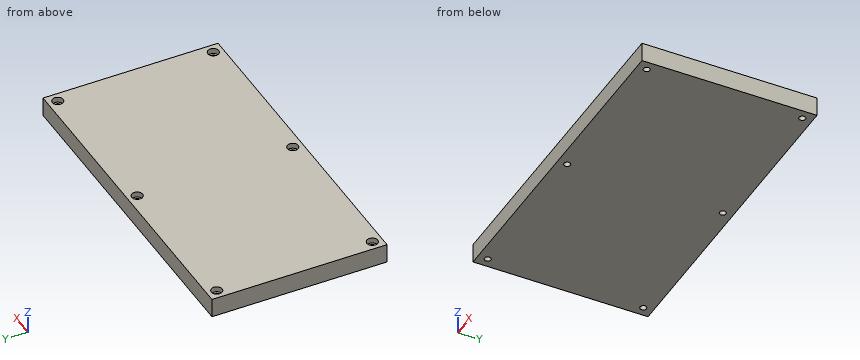
from build123d import *

# Parameters (mm, degrees)
SKETCH1_W                                      = 169.5
SKETCH1_H                                      = 90
BOSS_EXTRUDE1_DEPTH                            = 10
CBORE_FOR_4_SOCKET_HEAD_CAP_SCREW1_D           = 3.2639
CBORE_FOR_4_SOCKET_HEAD_CAP_SCREW1_CBORE_D     = 5.55752
CBORE_FOR_4_SOCKET_HEAD_CAP_SCREW1_CBORE_DEPTH = 2.8448


with BuildPart() as part:
    # Sketch1 → Boss-Extrude1 (new body)
    with BuildSketch(Plane.XY):
        with Locations((84.75, 45)):
            Rectangle(SKETCH1_W, SKETCH1_H)
    extrude(amount=BOSS_EXTRUDE1_DEPTH)

    # CBORE for #4 Socket Head Cap Screw1 (through all)
    with Locations(Plane.XY.offset(10)):
        with Locations((5, 85), (164.5, 85), (164.5, 5), (5, 5), (84.75, 5), (84.75, 85)):
            CounterBoreHole(CBORE_FOR_4_SOCKET_HEAD_CAP_SCREW1_D / 2, CBORE_FOR_4_SOCKET_HEAD_CAP_SCREW1_CBORE_D / 2, CBORE_FOR_4_SOCKET_HEAD_CAP_SCREW1_CBORE_DEPTH)


solid = part.part
Verification items for the finished model (mm, model axes). Coordinates: 2 decimals unless noted, no trailing zeros. Order: outer loops, then holes, each group sorted by start corner. A loop starts at its lowest first (then second) coordinate and runs counter-clockwise, first axis right, second up. Notation, with made-up numbers: M -9.5,10.25 L 25.5,10.25 A19 ccw 25.5,21.25 Z; hole C 6.5,24.25 d1. An arc over 180 degrees is marked long. One line per item, written item: value. Start each with the question number.
Item 1: Sectioned sample at B-B on y = 85. Record the cut outline in (x, z).
Item 2: Thickness scan on probe 1 along Y at (x, z) = (164.5, 9.4); probe 2 along Y at (x, z) = (164.5, 3). Record the ranges inside material, lowest first.
Item 3: Sectioned sample at A-A on x = 5. Record the cut outline in (y, z), then the cut area to 3 significant figures.
Item 4: Depth check by flat-ended pin: P1, Ø5, axis at x = 5, y = 5, coming from the +Z side. Enter the tip coordinate at first touch or a pass-through.
Calculated:
1. outline: M 0,0 L 3.37,0 L 3.37,7.16 L 2.22,7.16 L 2.22,10 L 0,10 Z; M 6.63,0 L 83.12,0 L 83.12,7.16 L 81.97,7.16 L 81.97,10 L 7.78,10 L 7.78,7.16 L 6.63,7.16 Z; M 86.38,0 L 162.87,0 L 162.87,7.16 L 161.72,7.16 L 161.72,10 L 87.53,10 L 87.53,7.16 L 86.38,7.16 Z; M 166.13,0 L 169.5,0 L 169.5,10 L 167.28,10 L 167.28,7.16 L 166.13,7.16 Z
2. probe 1: 0 to 2.22, 7.78 to 82.22, 87.78 to 90
2. probe 2: 0 to 3.37, 6.63 to 83.37, 86.63 to 90
3. outline: M 0,0 L 3.37,0 L 3.37,7.16 L 2.22,7.16 L 2.22,10 L 0,10 Z; M 6.63,0 L 83.37,0 L 83.37,7.16 L 82.22,7.16 L 82.22,10 L 7.78,10 L 7.78,7.16 L 6.63,7.16 Z; M 86.63,0 L 90,0 L 90,10 L 87.78,10 L 87.78,7.16 L 86.63,7.16 Z
3. area: 822 mm^2
4. P1: z = 7.16
